Check sheet for the modelled part. Datum: model origin and axes. Units: mm. A direction names the side the tool comes from. Give positions to 0.01 mm unless a question says otherwise; leave off trailing zeros. Loops run counter-clockwise (first coordinate to the right, second up) from the corner with the lowest first, then second, coordinate; pieces in that order, holes last. Notation, with made-up numbers: (72, 62.25) - (79, 62.25) arc R13 cw to (79, 78.25) - close; hole circle Ø7 at (-24, -22). An arc over 180 degrees is marked (long way). Use one line per item in the form item = value.
from build123d import *

# Parameters (mm, degrees)
SKETCH1_R           = 2.125
BOSS_EXTRUDE1_DEPTH = 100


with BuildPart() as part:
    # Sketch1 → Boss-Extrude1 (new body)
    with BuildSketch(Plane.XY):
        with BuildLine():
            Line((8.1, 5.225), (8.1, 2.85))
            Line((8.1, 2.85), (10, 4.75))
            Line((10, 4.75), (10, 8.5))
            ThreePointArc((10, 8.5), (9.560660172, 9.560660172), (8.5, 10))
            Line((8.5, 10), (4.75, 10))
            Line((4.75, 10), (2.85, 8.1))
            Line((2.85, 8.1), (5.225, 8.1))
            Line((5.225, 8.1), (5.225, 6.325))
            Line((5.225, 6.325), (2.9, 4))
            Line((2.9, 4), (-2.9, 4))
            Line((-2.9, 4), (-5.225, 6.325))
            Line((-5.225, 6.325), (-5.225, 8.1))
            Line((-5.225, 8.1), (-2.85, 8.1))
            Line((-2.85, 8.1), (-4.75, 10))
            Line((-4.75, 10), (-8.5, 10))
            ThreePointArc((-8.5, 10), (-9.560660172, 9.560660172), (-10, 8.5))
            Line((-10, 8.5), (-10, 4.75))
            Line((-10, 4.75), (-8.1, 2.85))
            Line((-8.1, 2.85), (-8.1, 5.225))
            Line((-8.1, 5.225), (-6.325, 5.225))
            Line((-6.325, 5.225), (-4, 2.9))
            Line((-4, 2.9), (-4, -2.9))
            Line((-4, -2.9), (-6.325, -5.225))
            Line((-6.325, -5.225), (-8.1, -5.225))
            Line((-8.1, -5.225), (-8.1, -2.85))
            Line((-8.1, -2.85), (-10, -4.75))
            Line((-10, -4.75), (-10, -8.5))
            ThreePointArc((-10, -8.5), (-9.560660172, -9.560660172), (-8.5, -10))
            Line((-8.5, -10), (-4.75, -10))
            Line((-4.75, -10), (-2.85, -8.1))
            Line((-2.85, -8.1), (-5.225, -8.1))
            Line((-5.225, -8.1), (-5.225, -6.325))
            Line((-5.225, -6.325), (-2.9, -4))
            Line((-2.9, -4), (2.9, -4))
            Line((2.9, -4), (5.225, -6.325))
            Line((5.225, -6.325), (5.225, -8.1))
            Line((5.225, -8.1), (2.85, -8.1))
            Line((2.85, -8.1), (4.75, -10))
            Line((4.75, -10), (8.5, -10))
            ThreePointArc((8.5, -10), (9.560660172, -9.560660172), (10, -8.5))
            Line((10, -8.5), (10, -4.75))
            Line((10, -4.75), (8.1, -2.85))
            Line((8.1, -2.85), (8.1, -5.225))
            Line((8.1, -5.225), (6.325, -5.225))
            Line((6.325, -5.225), (4, -2.9))
            Line((4, -2.9), (4, 2.9))
            Line((4, 2.9), (6.325, 5.225))
            Line((6.325, 5.225), (8.1, 5.225))
        make_face()
        Circle(SKETCH1_R, mode=Mode.SUBTRACT)
    extrude(amount=BOSS_EXTRUDE1_DEPTH)


solid = part.part
Item 1: Section check A-A on y = 7.25. Record the boundary of the cut face in (x, z) (3 decimals).
Answer block:
outline = (-10, 0) - (-5.225, 0) - (-5.225, 100) - (-10, 100) - close; (5.225, 0) - (10, 0) - (10, 100) - (5.225, 100) - close
Item 2: Section check B-B on x = 0. Record the boundary of the cut face in (y, z) (3 decimals), then the cut area to 3 significant figures.
Answer block:
outline = (-4, 0) - (-2.125, 0) - (-2.125, 100) - (-4, 100) - close; (2.125, 0) - (4, 0) - (4, 100) - (2.125, 100) - close
area = 375 mm2
Item 3: Access from +Z, -Z, +X, -X, +Y, -Y to the whole of each face (thin tool, end or side, straight path). Record for faces 1 (the face through (-5.1, -4, 49.3)), 2 (the face through (-9.04, -3.79, 49.3)), 3 (the face through (-3.81, -9.06, 49.3)).
Answer block:
face_1 = +Z, -Z
face_2 = +Z, -Z, -X
face_3 = +Z, -Z, -Y
Item 4: Gauge pin test, flat ends, axial feed: P1, Ø2.5, axis at x = 0, y = 0, coming from the +Z side; P2, Ø1.7, axis at x = 0.5, z = 59, coming from the -Y side; P3, Ø3, axis at y = 2, z = 81, coming from the -X side; P4, Ø4, axis at x = -5, y = 0.5, coming from the +Z side. Record the tip position at first contact, or that the pin passes through.
Answer block:
P1 = through
P2 = -4
P3 = -8.75
P4 = 100
Item 5: Thickness scan on L1, parallel to Y at x = 0, z = 66 (3 decimals); L2, parallel to X at y = 7.75, z = 45 (3 decimals); L3, parallel to Y at x = -2.75, z = 69.5. Record the ranges inside material, lowest first.
Answer block:
L1 = -4 to -2.125, 2.125 to 4
L2 = -10 to -5.225, 5.225 to 10
L3 = -4 to 4
Item 6: Mould release check, pull along X, two halves, no side actions. Record for faces 4 (the face through (-10, -7, 49)), 5 (the face through (5.225, 7, 49)): released by +X, released by -X, zero draft, split by the parting line, or undercut.
Answer block:
face_4 = released by -X
face_5 = undercut
